Could you check a few things on this model? Use its own coordinates, in mm. A direction names the side the tool comes from. Give positions to 0.01 mm unless a question says otherwise; leave off trailing zeros. Write each loop counter-clockwise with the first axis right and the second up, starting at its lowest first coordinate (ties: lowest second). Pieces come first, ordered by that corner, then holes. Notation, with made-up numbers: (12.5, -8) - (35.5, -8) arc R20 cw to (35.5, 31) - close; hole circle Ø6 at (-28, 60.25). An arc over 180 degrees is marked (long way). Write item = value, one per line.
from build123d import *

# Parameters (mm, degrees)
SKETCH1_R           = 25
SKETCH1_R_2         = 5
BOSS_EXTRUDE1_DEPTH = 20


with BuildPart() as part:
    # Sketch1 → Boss-Extrude1 (new body)
    with BuildSketch(Plane.XY):
        with BuildLine():
            Line((-60, 10), (-38.729833462, 10))
            ThreePointArc((-38.729833462, 10), (-34.641016151, 20), (-28.025170769, 28.541019662))
            Line((-28.025170769, 28.541019662), (-38.660254038, 46.961524227))
            ThreePointArc((-38.660254038, 46.961524227), (-35, 60.621778265), (-21.339745962, 56.961524227))
            Line((-21.339745962, 56.961524227), (-10.704662693, 38.541019662))
            ThreePointArc((-10.704662693, 38.541019662), (0, 40), (10.704662693, 38.541019662))
            Line((10.704662693, 38.541019662), (21.339745962, 56.961524227))
            ThreePointArc((21.339745962, 56.961524227), (35, 60.621778265), (38.660254038, 46.961524227))
            Line((38.660254038, 46.961524227), (28.025170769, 28.541019662))
            ThreePointArc((28.025170769, 28.541019662), (34.641016151, 20), (38.729833462, 10))
            Line((38.729833462, 10), (60, 10))
            ThreePointArc((60, 10), (70, 0), (60, -10))
            Line((60, -10), (38.729833462, -10))
            ThreePointArc((38.729833462, -10), (34.641016151, -20), (28.025170769, -28.541019662))
            Line((28.025170769, -28.541019662), (38.660254038, -46.961524227))
            ThreePointArc((38.660254038, -46.961524227), (35, -60.621778265), (21.339745962, -56.961524227))
            Line((21.339745962, -56.961524227), (10.704662693, -38.541019662))
            ThreePointArc((10.704662693, -38.541019662), (0, -40), (-10.704662693, -38.541019662))
            Line((-10.704662693, -38.541019662), (-21.339745962, -56.961524227))
            ThreePointArc((-21.339745962, -56.961524227), (-35, -60.621778265), (-38.660254038, -46.961524227))
            Line((-38.660254038, -46.961524227), (-28.025170769, -28.541019662))
            ThreePointArc((-28.025170769, -28.541019662), (-34.641016151, -20), (-38.729833462, -10))
            Line((-38.729833462, -10), (-60, -10))
            ThreePointArc((-60, -10), (-70, 0), (-60, 10))
        make_face()
        Circle(SKETCH1_R, mode=Mode.SUBTRACT)
        with Locations((-60, 0)):
            Circle(SKETCH1_R_2, mode=Mode.SUBTRACT)
        with Locations((-30, 51.961524227)):
            Circle(SKETCH1_R_2, mode=Mode.SUBTRACT)
        with Locations((30, 51.961524227)):
            Circle(SKETCH1_R_2, mode=Mode.SUBTRACT)
        with Locations((60, 0)):
            Circle(SKETCH1_R_2, mode=Mode.SUBTRACT)
        with Locations((30, -51.961524227)):
            Circle(SKETCH1_R_2, mode=Mode.SUBTRACT)
        with Locations((-30, -51.961524227)):
            Circle(SKETCH1_R_2, mode=Mode.SUBTRACT)
    extrude(amount=BOSS_EXTRUDE1_DEPTH)


solid = part.part
1. Which directions (+Z, -Z, +X, -X, +Y, -Y) give clear straight access to the entire face, cutting with the end or side of a thin tool? Please do faces 4 (the face through (-33.417, -37.88, 9.86)), 5 (the face through (16.097, -47.88, 9.86)), 6 (the face through (15.948, 47.622, 9.86)).
Filled sheet:
face_4 = +Z, -Z, -X
face_5 = +Z, -Z, -Y
face_6 = +Z, -Z, +Y
2. If we section it at D-D, the plane y = -18.5: Please give me the cut outline in (x, z).
Filled sheet:
outline = (-35.46, 0) - (-16.82, 0) - (-16.82, 20) - (-35.46, 20) - close; (16.82, 0) - (35.46, 0) - (35.46, 20) - (16.82, 20) - close
3. Thinking about a two-plate mould opening in X: for faces 1 (the face through (33.268, -37.622, 9.86)), 2 (the face through (23.846, 7.509, 9.86)), 3 (the face through (26, 0, 20)), which applies, pulls with the +X half, pulls with the -X half, needs draft (parallel to the pull), parting line crosses it, or undercut?
Filled sheet:
face_1 = pulls with the +X half
face_2 = undercut
face_3 = needs draft
4. If we section it at A-A, the plane y = 0: Please give me the cut outline in (x, z), and give its area (3 significant figures).
Filled sheet:
outline = (-70, 0) - (-65, 0) - (-65, 20) - (-70, 20) - close; (-55, 0) - (-25, 0) - (-25, 20) - (-55, 20) - close; (25, 0) - (55, 0) - (55, 20) - (25, 20) - close; (65, 0) - (70, 0) - (70, 20) - (65, 20) - close
area = 1,400 mm2
5. If we section it at C-C, the plane z = 9.5: Count the separate pieces of the cut face and the enclosed holes in it, and give its area (3 significant figures).
Filled sheet:
separate_pieces = 1
enclosed_holes = 7
area = 5,980 mm2
6. For pin 1 (2 mm diameter, centred on x = -3.5, y = 42, fed in from +Z); pin 2 (10 mm diameter, centred on y = 18, z = 9.5, fed in from +X); pin 3 (4 mm diameter, centred on x = 0.5, z = 13, fed in from +Y); pin 4 (10 mm diameter, centred on x = 51.5, z = 5.5, fed in from +Y), each with a flat end and sliding along its axis, tell me the tip position at first contact or that it passes through.
Filled sheet:
pin_1 = through
pin_2 = 37.83
pin_3 = 40
pin_4 = 10
7. If we section it at B-B, the plane x = 0: Please give me the cut outline in (y, z).
Filled sheet:
outline = (-40, 0) - (-25, 0) - (-25, 20) - (-40, 20) - close; (25, 0) - (40, 0) - (40, 20) - (25, 20) - close
8. I need wall thicknesses on line 1 (X direction, y = -48, z = 7.25); line 2 (X direction, y = -55.5, z = 16.25); line 3 (Y direction, x = 28.5, z = 9.75). Which ranges of each line are inside material? Lowest first, please.
Filled sheet:
line_1 = -39.18 to -33.05, -26.95 to -16.17, 16.17 to 26.95, 33.05 to 39.18
line_2 = -39.35 to -33.53, -26.47 to -20.5, 20.5 to 26.47, 33.53 to 39.35
line_3 = -61.85 to -56.73, -47.19 to -29.36, -28.07 to 28.07, 29.36 to 47.19, 56.73 to 61.85
